The listing builds one solid part. Answer for the finished solid, in the listing's coordinates (mm). A direction names the side the tool comes from. Give positions to 0.01 mm unless a question says otherwise; leave off trailing zeros. Write each loop counter-clockwise with the first axis right and the second up, starting at its lowest first coordinate (ties: lowest second). Pieces come first, ordered by that corner, then holes. Notation, with made-up numbers: (-30, 72.5) - (-3, 72.5) arc R37 cw to (-3, 108.5) - close; hole circle Ø7 at (4.25, -13.5). An arc over 180 degrees is marked (long way). Answer in a Markdown table with one row per item. Add a question column.
Autodesk Inventor part; units mm, degrees
ref_plane "Arbeitsebene1" through (0, 0, 7.4) normal (0, 0, 1) x (1, 0, 0)
ref_plane "YZ Plane" through (0, 0, 0) normal (1, 0, 0) x (0, 1, 0)
ref_plane "XZ Plane" through (0, 0, 0) normal (0, 1, 0) x (-1, 0, 0)
sketch "Skizze1" plane through (0, 0, 0) normal (0, 0, 1) x (1, 0, 0)
  line L0 (0, 1.75) -> (41.2, 1.75)
  line L1 (41.2, 1.75) -> (41.2, -1.75)
  line L2 (41.2, -1.75) -> (0, -1.75)
  line L3 (0, -1.75) -> (0, 1.75)
  point P0 (0, 0)
  point P1 (0, 0)
  dimension "d0" = 41.2
  dimension "d1" = 3.5
extrude "Extrusion1" add sketch "Skizze1" along normal blind 14.8
sketch "Skizze2" plane through (0, 0, 0) normal (0, 0, -1) x (-1, 0, 0)
  line L0 (0, 0) -> (-3, 0) construction
  line L1 (-3, 0) -> (-32, 0) construction
  dimension "d4" = 3
  dimension "d5" = 32
hole "Bohrung1" at (3, 0, 0) at (32, 0, 0) direction (0, 0, 1) diameter 2.013 depth 9 tip angle 118
sketch "Skizze3" plane through (0, 0, 0) normal (0, 0, -1) x (-1, 0, 0)
  circle A0 centre (-3, 0) radius 1.0065
  circle A1 centre (-32, 0) radius 1.0065
  line L0 (0, 1.75) -> (-41.2, 1.75)
  line L1 (-41.2, 1.75) -> (-41.2, -1.75)
  line L2 (-41.2, -1.75) -> (0, -1.75)
  line L3 (0, -1.75) -> (0, 1.75)
  line L4 (-41.2, -1.75) -> (0, -1.75)
  line L5 (-9, -1.75) -> (-17, -1.75)
  line L6 (-17, -1.75) -> (-17, 1.75)
  line L7 (-17, 1.75) -> (-9, 1.75)
  line L8 (-9, 1.75) -> (-9, -1.75)
  line L9 (-17, 0) -> (-9, 0) construction
  point P0 (0, 0)
  point P1 (-13, 0)
  dimension "d13" = 13
  dimension "d14" = 8
extrude "Extrusion2" cut sketch "Skizze3" against normal blind 1 contours L8 L2 L6 L0
sketch "Skizze4" plane through (41.2, -1.75, 0) normal (1, 0, 0) x (0, 0, -1)
  line L0 (0, 1.75) -> (-3.5, 1.75) construction
  line L1 (-3.5, 1.75) -> (-11.5, 1.75) construction
  dimension "d17" = 3.5
  dimension "d19" = 8
hole "Bohrung2" at (41.2, 0, 11.5) at (41.2, 0, 3.5) direction (-1, 0, 0) diameter 2.013 depth 7 tip angle 118
ref_plane "Arbeitsebene1" through (0, 0, 7.4) normal (0, 0, 1) x (1, 0, 0)
properties part number "USB Wärmeableiter 1"
1. Section A-A (z = 1.75) is taken. Give the vertices of the cut face in (x, y).
2. Given pin 1 Ø1.2 at (x, y) = (32, 0) entering from -Z, flat-ended and moving along its own axis, determine where the tip first touches the part or whether it passes through.
3. Straight lines are drawn through the part: L1, parallel to Z at x = 35.75, y = 0; L2, parallel to X at y = 0, z = 6.5; L3, parallel to Y at x = 3, z = 1.25. For each, find the intervals that lie inside material, in ascending order. Write a range as [from, to].
4. The mould has two halves that part along X. Classify faces 1 (the face through (20, 1.75, 7)), 2 (the face through (17, 0, 0.5)), 3 (the face through (33.7, 0.05, 3.33)), 4 (the face through (0, 0, 7)): +X half, -X half, draft (parallel to the pull), parting line (faces both ways), or undercut.
5. A tool of negligible diameter and unlimited length cuts with its end or side. For faces 5 (the face through (37.651, -0.044, 4.506)), 6 (the face through (29, 0, 0)), 7 (the face through (3.983, -0.218, 4.563)), 8 (the face through (9, 0, 0.5)), 9 (the face through (21, -1.75, 7)), from which of +Z, -Z, +X, -X, +Y, -Y can it reach the whole face along a straight path? Write none if from no direction.
6. Section B-B (x = 14.5) is taken. Give the vertices of the cut face in (y, z), and give its area (3 significant figures).
Geometry check:
| question | item | result |
|---|---|---|
| 1 | outline | (0, -1.75) - (41.2, -1.75) - (41.2, 1.75) - (0, 1.75) - close; hole circle Ø2.01 at (3, 0); hole circle Ø2.01 at (32, 0) |
| 2 | pin 1 | z = 9.24 |
| 3 | L1 | [0, 2.49], [4.51, 10.49], [12.51, 14.8] |
| 3 | L2 | [0, 1.99], [4.01, 30.99], [33.01, 41.2] |
| 3 | L3 | [-1.75, -1.01], [1.01, 1.75] |
| 4 | face 1 | draft |
| 4 | face 2 | undercut |
| 4 | face 3 | +X half |
| 4 | face 4 | -X half |
| 5 | face 5 | +X |
| 5 | face 6 | -Z, +X, -X, +Y, -Y |
| 5 | face 7 | -Z |
| 5 | face 8 | -Z, +Y, -Y |
| 5 | face 9 | +Z, -Z, +X, -X, -Y |
| 6 | outline | (-1.75, 1) - (1.75, 1) - (1.75, 14.8) - (-1.75, 14.8) - close |
| 6 | area | 48.3 mm² |
